from build123d import *

# Parameters (mm, degrees)
EXTRUDE_1_DEPTH     = 5
SKETCH_5_R          = 21.15
CUT_EXTRUDE_1_DEPTH = 3
SKETCH_6_R          = 4
CUT_EXTRUDE_2_DEPTH = 37
SKETCH_7_R          = 1.8
CUT_EXTRUDE_3_DEPTH = 37
CUT_EXTRUDE_4_DEPTH = 12
CHAMFER_1_SIZE      = 2


with BuildPart() as part:
    # 草图1 → 凸台-拉伸1 (new body)
    with BuildSketch(Plane.XY):
        Polygon((24, 35.52), (35.52, 24), (35.52, -24), (24, -35.52), (24, -77.52), (-24, -77.52), (-24, -35.52), (-35.52, -24), (-35.52, 24), (-24, 35.52), align=None)
        with BuildLine():
            Line((11.2, -54.52), (11.2, -58.52))
            ThreePointArc((11.2, -58.52), (0, -69.72), (-11.2, -58.52))
            Line((-11.2, -58.52), (-11.2, -54.52))
            ThreePointArc((-11.2, -54.52), (0, -43.32), (11.2, -54.52))
        make_face(mode=Mode.SUBTRACT)
        with BuildLine():
            Line((-17.15, -42.52), (-17.15, -39.52))
            ThreePointArc((-17.15, -39.52), (-15.5, -37.87), (-13.85, -39.52))
            Line((-13.85, -39.52), (-13.85, -42.52))
            ThreePointArc((-13.85, -42.52), (-15.5, -44.17), (-17.15, -42.52))
        make_face(mode=Mode.SUBTRACT)
        with BuildLine():
            Line((17.15, -42.52), (17.15, -39.52))
            ThreePointArc((17.15, -39.52), (15.5, -37.87), (13.85, -39.52))
            Line((13.85, -39.52), (13.85, -42.52))
            ThreePointArc((13.85, -42.52), (15.5, -44.17), (17.15, -42.52))
        make_face(mode=Mode.SUBTRACT)
        with BuildLine():
            Line((17.15, -70.52), (17.15, -73.52))
            ThreePointArc((17.15, -73.52), (15.5, -75.17), (13.85, -73.52))
            Line((13.85, -73.52), (13.85, -70.52))
            ThreePointArc((13.85, -70.52), (15.5, -68.87), (17.15, -70.52))
        make_face(mode=Mode.SUBTRACT)
        with BuildLine():
            Line((-17.15, -70.52), (-17.15, -73.52))
            ThreePointArc((-17.15, -73.52), (-15.5, -75.17), (-13.85, -73.52))
            Line((-13.85, -73.52), (-13.85, -70.52))
            ThreePointArc((-13.85, -70.52), (-15.5, -68.87), (-17.15, -70.52))
        make_face(mode=Mode.SUBTRACT)
    extrude(amount=EXTRUDE_1_DEPTH)

    # 草图3 → 放样1 section 0
    with BuildSketch(Plane.XY.offset(15)):
        with BuildLine():
            Line((11.183766184, 27), (-11.183766184, 27))
            Line((-11.183766184, 27), (-27, 11.183766184))
            Line((-27, 11.183766184), (-27, -11.183766184))
            Line((-27, -11.183766184), (-11.183766184, -27))
            Line((-11.183766184, -27), (11.183766184, -27))
            Line((11.183766184, -27), (27, -11.183766184))
            Line((27, -11.183766184), (27, 11.183766184))
            Line((27, 11.183766184), (11.183766184, 27))
        make_face()
    # 草图4 → 放样1 section 1
    with BuildSketch(Plane.XY.offset(5)):
        with BuildLine():
            Line((-24, -35.52), (24, -35.52))
            Line((24, -35.52), (35.52, -24))
            Line((35.52, -24), (35.52, 24))
            Line((35.52, 24), (24, 35.52))
            Line((24, 35.52), (-24, 35.52))
            Line((-24, 35.52), (-35.52, 24))
            Line((-35.52, 24), (-35.52, -24))
            Line((-35.52, -24), (-24, -35.52))
        make_face()
    loft()

    # 草图5 → 切除-拉伸1 (cut)
    with BuildSketch(Plane.XY.offset(15)):
        Circle(SKETCH_5_R)
    extrude(amount=-CUT_EXTRUDE_1_DEPTH, mode=Mode.SUBTRACT)

    # 草图6 → 切除-拉伸2 (cut)
    with BuildSketch(Plane.XY.offset(12)):
        Circle(SKETCH_6_R)
    extrude(amount=-CUT_EXTRUDE_2_DEPTH, mode=Mode.SUBTRACT)

    # 草图7 → 切除-拉伸3 (cut)
    with BuildSketch(Plane(origin=(0, 0, 0), x_dir=(-1, 0, 0), z_dir=(0, 0, -1))):
        with Locations((29.12, 15)):
            Circle(SKETCH_7_R)
        with Locations(Location((29.12, -15, 0), (0, 0, 314.737833249))):
            Circle(SKETCH_7_R)
        with Locations((-29.12, -15)):
            Circle(SKETCH_7_R)
        with Locations(Location((-29.12, 15, 0), (0, 0, 292.492646576))):
            Circle(SKETCH_7_R)
        with Locations((-15, 29.12)):
            Circle(SKETCH_7_R)
        with Locations(Location((15, 29.12, 0), (0, 0, 44.737833249))):
            Circle(SKETCH_7_R)
    extrude(amount=-CUT_EXTRUDE_3_DEPTH, mode=Mode.SUBTRACT)

    # 草图8 → 切除-拉伸4 (cut)
    with BuildSketch(Plane.XY.offset(15)):
        Polygon((-29.12, -11.535898385), (-32.12, -13.267949192), (-32.12, -16.732050808), (-29.12, -18.464101615), (-26.12, -16.732050808), (-26.12, -13.267949192), align=None)
        Polygon((-26.12, 13.267949192), (-29.12, 11.535898385), (-32.12, 13.267949192), (-32.12, 16.732050808), (-29.12, 18.464101615), (-26.12, 16.732050808), align=None)
        Polygon((13.267949192, 26.12), (11.535898385, 29.12), (13.267949192, 32.12), (16.732050808, 32.12), (18.464101615, 29.12), (16.732050808, 26.12), align=None)
        Polygon((-11.535898385, 29.12), (-13.267949192, 32.12), (-16.732050808, 32.12), (-18.464101615, 29.12), (-16.732050808, 26.12), (-13.267949192, 26.12), align=None)
        Polygon((26.12, -13.267949192), (29.12, -11.535898385), (32.12, -13.267949192), (32.12, -16.732050808), (29.12, -18.464101615), (26.12, -16.732050808), align=None)
        Polygon((29.12, 11.535898385), (32.12, 13.267949192), (32.12, 16.732050808), (29.12, 18.464101615), (26.12, 16.732050808), (26.12, 13.267949192), align=None)
    extrude(amount=-CUT_EXTRUDE_4_DEPTH, mode=Mode.SUBTRACT)

    # 倒角1
    chamfer_1_edges = [part.edges().sort_by_distance(p)[0] for p in [
        (24, -77.52, 2.5),
        (-24, -77.52, 2.5),
    ]]
    chamfer(chamfer_1_edges, length=CHAMFER_1_SIZE)


solid = part.part
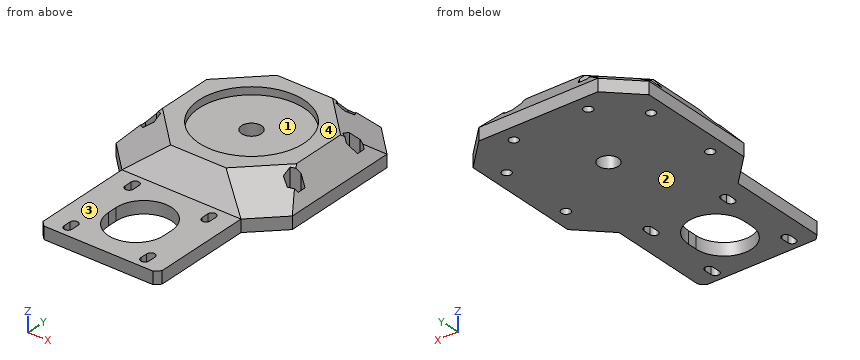
Input: part model. Units: mm. Frame: model coordinates. Face numbers are marked on the shaded views. A direction names the side the tool comes from. Give positions to 0.01 mm unless a question says otherwise; leave off trailing zeros. Order: outer loops, then holes, each group sorted by start corner. A loop starts at its lowest first (then second) coordinate and runs counter-clockwise, first axis right, second up.
Q1. Contact query for flat-ended pins moving along their axis: pin 1 Ø3 at (x, y) = (-30.5, 15) entering from +Z; pin 2 Ø0.9 at (y, z) = (-40.5, 2) entering from +X; pin 3 Ø10 at (x, y) = (-26.5, 22.5) entering from +Z; pin 4 Ø6 at (x, y) = (25, -47) entering from -Z. Output: stop coordinate, or through.
Checked values:
pin 1: stops at z = 3
pin 2: stops at x = 24
pin 3: stops at z = 13.24
pin 4: stops at z = 0
Q2. Section B-B on x = 0. State how many separate pieces and enclosed holes the cut face has, and give its area (4 significant figures).
Checked values:
separate pieces: 3
enclosed holes: 0
area: 835.5 mm2
Q3. Set-up query: the marked faces 3 and 4. Return all of +Z, -Z, +X, -X, +Y, -Y with unobstructed straight access to the full face (end or side cutting, diameter ignored); none if empty.
Checked values:
face 3: +Z, +X, -X, -Y
face 4: +Z, +X, -X, +Y, -Y
Q4. Draft query along Y for the marked faces 1 and 2. Return one class per face: +Y half, -Y half, draft (parallel to the pull), parting line (faces both ways), or undercut.
Checked values:
face 1: undercut
face 2: draft
Q5. Section A-A on y = -47. Output: boundary loops of the cut face in (x, z).
Checked values:
outline: (-24, 0) - (-8.3, 0) - (-8.3, 5) - (-24, 5) - close; (8.3, 0) - (24, 0) - (24, 5) - (8.3, 5) - close
Q6. Ray query, probe 1 along X at (y, z) = (-16.5, 1.75); probe 2 along Y at (x, z) = (-30.5, 5.75); probe 3 along Y at (x, z) = (-27.5, 5.25). Return the intervals inside material, ascending.
Checked values:
probe 1: x = -35.52 to -30.11, -28.13 to 28.13, 30.11 to 35.52
probe 2: y = -27.42 to -17.67, -12.33 to 12.33, 17.67 to 27.42
probe 3: y = -31.49 to -17.53, -12.47 to 12.47, 17.53 to 31.49
